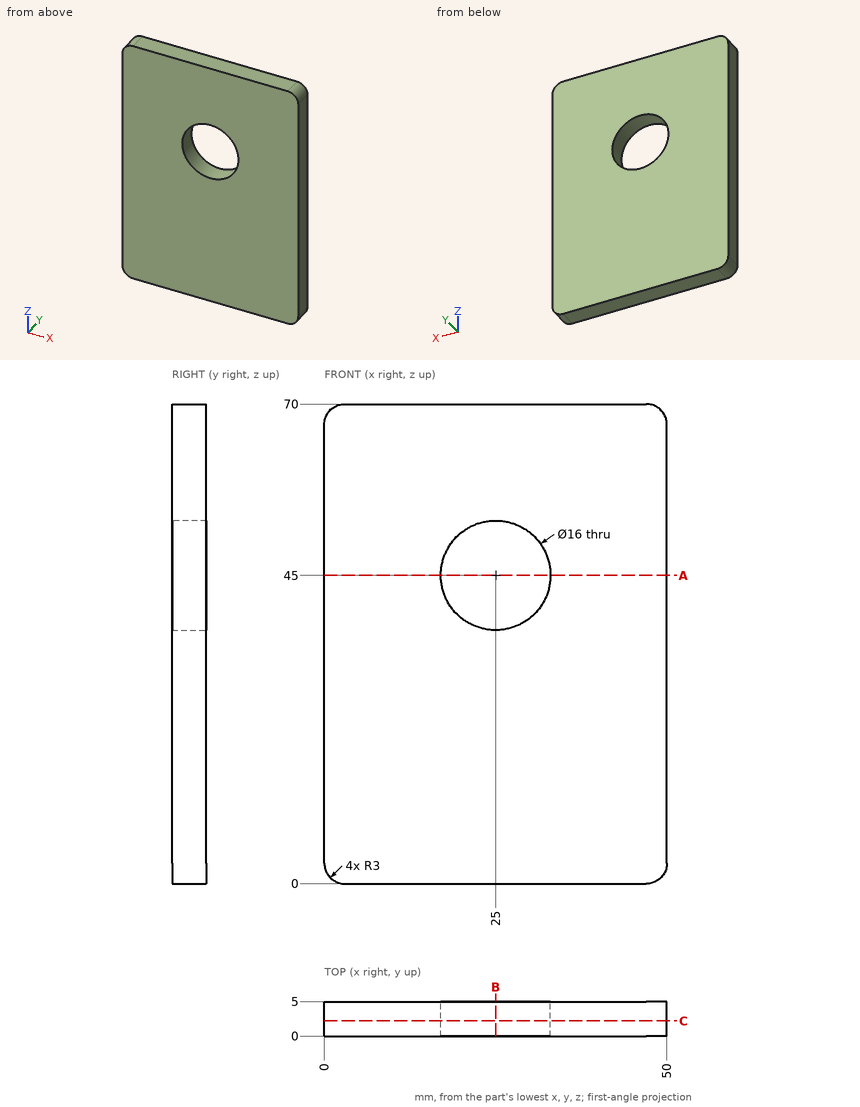
Geometry: see drawing. Coordinates: mm, zero at the bounding-box minimum. Round coordinates to 2 decimals unless told otherwise and drop trailing zeros. Loops run counter-clockwise (first coordinate to the right, second up) from the corner with the lowest first, then second, coordinate; pieces in that order, holes last. Notation, with made-up numbers: (65, -23) -> (96, -23) arc R24 cw to (96, 2) -> close; hole circle Ø2 at (46.5, -4.5). An arc over 180 degrees is marked (long way). Write each question's results on one line, items separated by ' | '.
Item 1: Pin query (flat end, axial travel): pin 1 Ø8 at (x, z) = (31, 47) entering from -Y. Return the tip coordinate at first contact, or that it passes through.
Answers below:
pin 1: stops at y = 0
Item 2: Line query: probe 1 along X at (y, z) = (1.5, 45); probe 2 along Z at (x, y) = (30.5, 3.85); probe 3 along Z at (x, y) = (22.5, 4.35). Output: solid intervals per line, ascending. Write a range as [from, to].
Answers below:
probe 1: x = [0, 17], [33, 50] | probe 2: z = [0, 39.19], [50.81, 70] | probe 3: z = [0, 37.4], [52.6, 70]
Item 3: Cut plane B-B on x = 25. Return the cut outline in (y, z), and give its area (3 significant figures).
Answers below:
outline: (0, 0) -> (5, 0) -> (5, 37) -> (0, 37) -> close; (0, 53) -> (5, 53) -> (5, 70) -> (0, 70) -> close | area: 270 mm²
Item 4: Cut plane C-C on y = 2.2. Return the cut outline in (x, z), and give its area (3 significant figures).
Answers below:
outline: (0, 3) arc R3 ccw to (3, 0) -> (47, 0) arc R3 ccw to (50, 3) -> (50, 67) arc R3 ccw to (47, 70) -> (3, 70) arc R3 ccw to (0, 67) -> close; hole circle Ø16 at (25, 45) | area: 3,290 mm²
Item 5: Cut plane A-A on z = 45. Return the cut outline in (x, y).
Answers below:
outline: (0, 0) -> (17, 0) -> (17, 5) -> (0, 5) -> close; (33, 0) -> (50, 0) -> (50, 5) -> (33, 5) -> close
